Geometry: final body of the model. Coordinates: model frame, mm. A direction names the side the tool comes from. Round coordinates to 2 decimals unless told otherwise and drop trailing zeros. Loops run counter-clockwise (first coordinate to the right, second up) from the corner with the lowest first, then second, coordinate; pieces in that order, holes last. Notation, with made-up numbers: (23, 82) - (58, 82) arc R12 cw to (58, 90) - close; hole circle Ø7 at (13.25, -8.5). An arc over 180 degrees is marked (long way). Write item = value, one per line. Start each with the question number.
Item 1: First-contact query: pin 1 (2 mm diameter, centred on x = -8.5, z = 15.5, fed in from -Y); pin 2 (5 mm diameter, centred on x = -11.5, z = 5.5, fed in from -Y). Flat tips, straight axial feed; report the tip coordinate or a pass-through.
Item 2: Access query for faces 1 (the cylindrical face through (-14.985, 0.66, 10.647)), 2 (the flat face through (13, 8, 21)). Directions: +Z, -Z, +X, -X, +Y, -Y. A direction counts if a zero-diameter tool reaches every point of the face in a straight line with its end or side. Return the directions, or none.
Item 3: Section C-C (z = 22). Return loops of the section in (x, y).
Item 4: Section D-D (z = 7.75). Return loops of the section in (x, y), plus the area to 3 significant figures.
Item 5: Line query: line 1 (Y direction, x = 0, z = 9.75); line 2 (X direction, y = 0.5, z = 17.5); line 3 (Y direction, x = 0, z = 21.7). Output: solid intervals per line, ascending. Write a range as from..to.
Item 6: Section A-A (x = 0). Return loops of the section in (y, z).
Item 7: Draft query along Y for faces 3 (the flat face through (0, 20, 0)), 4 (the cylindrical face through (-13.887, -10.648, 22.521)), 5 (the flat face through (0, 37, 12)), 6 (the cylindrical face through (0.55, -24.994, 11.832)). Return one class per face: pulls with the +Y half, pulls with the -Y half, needs draft (parallel to the pull), parting line crosses it, or undercut.
Item 8: Section B-B (y = 7). Return loops of the section in (x, z), plus the area to 3 significant figures.
from build123d import *

# Parameters (mm, degrees)
EXTRUDE_1_DEPTH     = 24
SKETCH_2_R          = 17.5
CUT_EXTRUDE_1_DEPTH = 3
CUT_EXTRUDE_2_REACH = 51.346
SKETCH_3_R          = 15


with BuildPart() as part:
    # 草图1 → 凸台-拉伸1 (new body)
    with BuildSketch(Plane.XY):
        with BuildLine():
            Line((-25, 0), (-25, 37))
            Line((-25, 37), (25, 37))
            Line((25, 37), (25, 0))
            ThreePointArc((25, 0), (0, -25), (-25, 0))
        make_face()
    extrude(amount=EXTRUDE_1_DEPTH)

    # 草图2 → 切除-拉伸1 (cut)
    with BuildSketch(Plane.XY.offset(24)):
        Circle(SKETCH_2_R)
    extrude(amount=-CUT_EXTRUDE_1_DEPTH, mode=Mode.SUBTRACT)

    # 草图3 → 切除-拉伸2 (cut, up to next)
    with BuildSketch(Plane.XY.offset(21), mode=Mode.PRIVATE) as cut_extrude_2_sk1:
        Circle(SKETCH_3_R)
    cut_extrude_2_tool1 = extrude(cut_extrude_2_sk1.sketch, amount=-CUT_EXTRUDE_2_REACH, mode=Mode.PRIVATE) & part.part
    add(cut_extrude_2_tool1.solids().sort_by_distance((0, 0, 21))[0], mode=Mode.SUBTRACT)


solid = part.part
Taken from the geometry:
q1.pin_1 = -23.85
q1.pin_2 = -23.32
q2.face_1 = +Z, -Z
q2.face_2 = +Z
q3.outline = (-25, 0) arc R25 ccw to (25, 0) - (25, 37) - (-25, 37) - close; hole circle Ø35 at (0, 0)
q4.outline = (-25, 0) arc R25 ccw to (25, 0) - (25, 37) - (-25, 37) - close; hole circle Ø30 at (0, 0)
q4.area = 2,120 mm^2
q5.line_1 = -25..-15, 15..37
q5.line_2 = -25..-14.99, 14.99..25
q5.line_3 = -25..-17.5, 17.5..37
q6.outline = (-25, 0) - (-15, 0) - (-15, 21) - (-17.5, 21) - (-17.5, 24) - (-25, 24) - close; (15, 0) - (37, 0) - (37, 24) - (17.5, 24) - (17.5, 21) - (15, 21) - close
q7.face_3 = needs draft
q7.face_4 = undercut
q7.face_5 = pulls with the +Y half
q7.face_6 = pulls with the -Y half
q8.outline = (-25, 0) - (-13.27, 0) - (-13.27, 21) - (-16.04, 21) - (-16.04, 24) - (-25, 24) - close; (13.27, 0) - (25, 0) - (25, 24) - (16.04, 24) - (16.04, 21) - (13.27, 21) - close
q8.area = 547 mm^2
